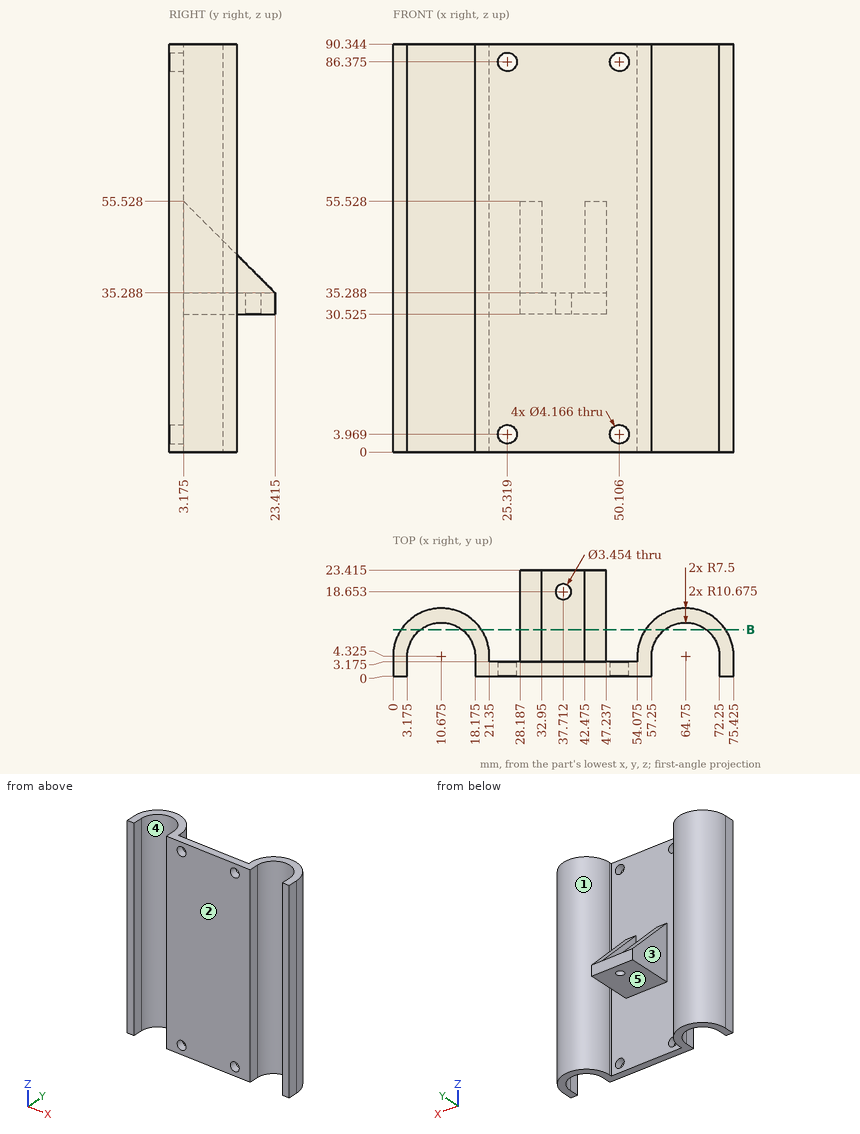
Print and shaded views of the part. All mm, measured from the part's lowest x, y and z. A direction names the side the tool comes from. Coordinates: 2 decimals unless noted, no trailing zeros.
Item 1: Drill centre lines: L1, parallel to X at y = 4.75, z = 13.5; L2, parallel to Y at x = 47, z = 78.5 (1 decimal); L3, parallel to X at y = 8, z = 23 (1 decimal). Where is each one in solid material? Low to high.
Filled in:
L1: x = 0.01 to 3.19, 18.16 to 21.34, 54.08 to 57.26, 72.24 to 75.42
L2: y = 0 to 3.2
L3: x = 0.7 to 4.1, 17.2 to 20.7, 54.7 to 58.2, 71.3 to 74.8
Item 2: Drop flat-ended pins along their axis: pin 1 Ø10 at (y, z) = (11, 48.5) entering from -X; pin 2 Ø1.5 at (y, z) = (13.5, 31.5) entering from +X (1 decimal); pin 3 Ø10 at (y, z) = (15, 64) entering from -X. Give the stop position or say it passes through.
Filled in:
pin 1: stops at x = 0.13
pin 2: stops at x = 71.3
pin 3: stops at x = 1.63
Item 3: Tool access for the marked faces 3, 4 and 5: list every direction of +Z, -Z, +X, -X, +Y, -Y with a clear straight run to the whole face (end or side of a thin tool).
Filled in:
face 3: +Z, -Z, +Y
face 4: +Z, -Z, -Y
face 5: -Z, +Y
Item 4: Mould opens along X. For the marked faces 1 and 2 say: released by +X, released by -X, zero draft, split by the parting line, or undercut.
Filled in:
face 1: undercut
face 2: zero draft
Item 5: Saw through at B-B on y = 10.25. State how many separate pieces and enclosed holes the cut face has, then the cut area to 3 significant figures.
Filled in:
separate pieces: 5
enclosed holes: 0
area: 1,760 mm2
